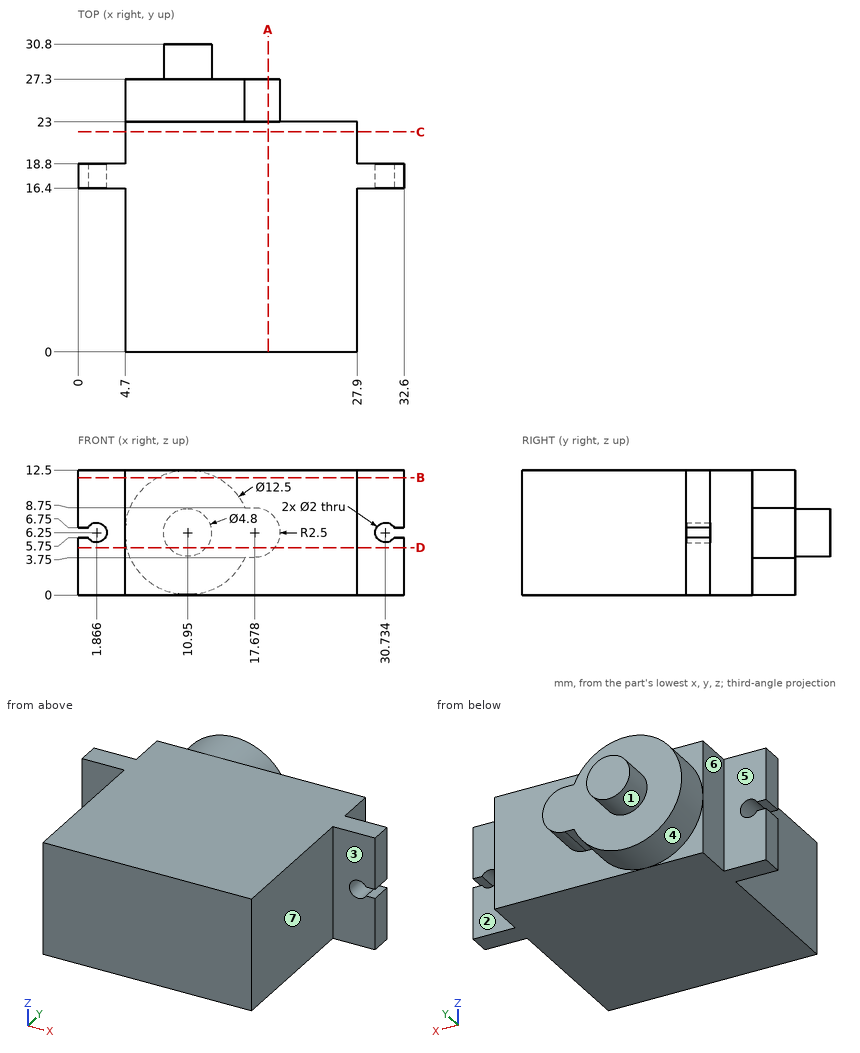
Can you work these out from the drawing? Everything is in mm from the part's minimum corner. A direction names the side the tool comes from. Coordinates: 2 decimals unless noted, no trailing zeros. Order: outer loops, then holes, each group sorted by start corner. A loop starts at its lowest first (then second) coordinate and runs counter-clockwise, first axis right, second up. Notation, with made-up numbers: M 44.25,77.5 L 80.25,77.5 A17 cw 80.25,95.5 Z; hole C -39.5,40.5 d6. An arc over 180 degrees is marked long. Answer as CSV lines item,"result". Start each with the question number.
1. I want a section at D-D, the plane z = 4.75. Write out the boundary of the cut face in (x, y), and give its area (3 significant figures).
2. We'd pull the mould along X, two halves only. Please class the marked faces 4, 5, 6 and 7: released by +X, released by -X, zero draft, split by the parting line, or undercut.
3. I want a section at C-C, the plane y = 22. Write out the boundary of the cut face in (x, z), and give its area (3 significant figures).
4. For pin 1 (4 mm diameter, centred on x = 2.5, z = 5, fed in from -Y); pin 2 (6 mm diameter, centred on y = 9, z = 4.5, fed in from -X); pin 3 (4 mm diameter, centred on x = 13, y = 24.5, fed in from +Z); pin 4 (1.5 mm diameter, centred on y = 6, z = 10.5, fed in from +X), each with a flat end and sliding along its axis, tell me the tip position at first contact or that it passes through.
5. I want a section at A-A, the plane x = 19. Write out the boundary of the cut face in (y, z).
6. On a 3-axis mill with a long thin cutter (end or side, diameter ignored), from which of +Z, -Z, +X, -X, +Y, -Y can I reach the whole of each face in a straight line? I mean the marked faces 1, 2 and 3. Say none if no direction works.
7. I need wall thicknesses on line 1 (X direction, y = 17.95, z = 6.25); line 2 (X direction, y = 21, z = 11.75); line 3 (Y direction, x = 13.5, z = 7.5). Which ranges of each line are inside material? Lowest first, please. Write a range as [from, to].
8. I want a section at B-B, the plane z = 11.75. Write out the boundary of the cut face in (x, y).
Recorded:
1,outline,"M 0,16.4 L 4.7,16.4 L 4.7,0 L 27.9,0 L 27.9,16.4 L 32.6,16.4 L 32.6,18.8 L 27.9,18.8 L 27.9,23 L 19.68,23 L 19.68,27.3 L 12.82,27.3 L 12.82,30.8 L 9.08,30.8 L 9.08,27.3 L 4.88,27.3 L 4.88,23 L 4.7,23 L 4.7,18.8 L 0,18.8 Z"
1,area,"633 mm2"
2,face 4,"split by the parting line"
2,face 5,"zero draft"
2,face 6,"released by -X"
2,face 7,"released by +X"
3,outline,"M 4.7,0 L 27.9,0 L 27.9,12.5 L 4.7,12.5 Z"
3,area,"290 mm2"
4,pin 1,"stops at y = 16.4"
4,pin 2,"stops at x = 4.7"
4,pin 3,"stops at z = 12.5"
4,pin 4,"stops at x = 27.9"
5,outline,"M 0,0 L 23,0 L 23,4.13 L 27.3,4.13 L 27.3,8.37 L 23,8.37 L 23,12.5 L 0,12.5 Z"
6,face 1,"+Y"
6,face 2,"+Z, -Z, +X, +Y"
6,face 3,"+Z, -Z, +X, -Y"
7,line 1,"x = [2.87, 29.73]"
7,line 2,"x = [4.7, 27.9]"
7,line 3,"y = [0, 27.3]"
8,outline,"M 0,16.4 L 4.7,16.4 L 4.7,0 L 27.9,0 L 27.9,16.4 L 32.6,16.4 L 32.6,18.8 L 27.9,18.8 L 27.9,23 L 13.92,23 L 13.92,27.3 L 7.98,27.3 L 7.98,23 L 4.7,23 L 4.7,18.8 L 0,18.8 Z"
